Read the model definition and answer for the solid it produces. Units are mm, in the model's axes. Coordinates: 2 decimals unless noted, no trailing zeros. Order: outer loops, then holes, each group sorted by start corner. A loop starts at its lowest first (then second) coordinate and runs counter-clockwise, first axis right, second up. Notation, with made-up numbers: (-15, 21) - (2, 21) arc R21 ccw to (2, 34) - close; hole circle Ø3 at (74, 81). An arc over 180 degrees is marked (long way). Use one line per item in the form item = value.
Autodesk Inventor part; units mm, degrees
ref_plane "Work Plane1" through (0, 12, 0) normal (0, 1, 0) x (-1, 0, 0)
ref_plane "YZ Plane" through (0, 0, 0) normal (1, 0, 0) x (0, 1, 0)
ref_plane "XY Plane" through (0, 0, 0) normal (0, 0, 1) x (1, 0, 0)
sketch "Sketch1" plane through (0, 0, 0) normal (0, 0, 1) x (1, 0, 0)
  arc A0 (0, -12) -> (0, 12) centre (0, 0) ccw
  line L0 (0, 12) -> (0, -12)
  dimension "d0" = 24
revolve "Revolution1" add sketch "Sketch1" angle 360 about axis through (0, 12, 0) along (0, -1, 0)
sketch "Sketch2" plane through (0, 0, 0) normal (0, 1, 0) x (-1, 0, 0)
  circle A0 centre (0, 0) radius 3.175
  dimension "d2" = 6.35
extrude "Extrusion1" cut sketch "Sketch2" along normal through all both and the other way through all
ref_plane "Work Plane1" through (0, 12, 0) normal (0, 1, 0) x (-1, 0, 0)
sketch "Sketch3" plane through (0, 12, 0) normal (0, 1, 0) x (-1, 0, 0)
  circle A0 centre (0, 0) radius 12
extrude "Extrusion2" cut sketch "Sketch3" against normal blind 3
mirror "Mirror1" about plane through (0, 0, 0) normal (0, 1, 0) of "Extrusion2"
properties part number "shifter ball"
(1) Section D-D, the plane z = -9 is taken. Write down the section's boundary in (x, y).
Answer list:
outline = circle Ø15.87 at (0, 0)
(2) Section C-C, the plane y = -1.75 is taken. Write down the section's boundary in (x, z) (3 decimals), then the cut area to 3 significant figures.
Answer list:
outline = circle Ø23.743 at (0, 0); hole circle Ø6.35 at (0, 0)
area = 411 mm2
(3) The mould has two halves that part along Z. Classify faces 1 (the flat face through (3.4, -9, 0.1)), 2 (the cylindrical face through (0.69, 0.13, -3.1)): +Z half, -Z half, draft (parallel to the pull), parting line (faces both ways), or undercut.
Answer list:
face_1 = draft
face_2 = undercut
(4) Section A-A, the plane x = 0 is taken. Write down the section's boundary in (y, z) (3 decimals).
Answer list:
outline = (-9, -7.937) arc R12 ccw to (9, -7.937) - (9, -3.175) - (-9, -3.175) - close; (-9, 3.175) - (9, 3.175) - (9, 7.937) arc R12 ccw to (-9, 7.937) - close
(5) Straight lines are drawn through the part: L1, parallel to X at y = 2.75, z = 2.25; L2, parallel to Z at x = 0, y = 4.5 (3 decimals); L3, parallel to Z at x = 1.75, y = -2. For each, find the intervals that lie inside material, in ascending order.
Answer list:
L1 = -11.46 to -2.24, 2.24 to 11.46
L2 = -11.124 to -3.175, 3.175 to 11.124
L3 = -11.7 to -2.65, 2.65 to 11.7
(6) Section B-B, the plane z = 0 is taken. Write down the section's boundary in (x, y) (3 decimals).
Answer list:
outline = (-7.937, -9) - (-3.175, -9) - (-3.175, 9) - (-7.937, 9) arc R12 ccw to start; (3.175, -9) - (7.937, -9) arc R12 ccw to (7.937, 9) - (3.175, 9) - close
(7) Given pin 1 Ø10 at (y, z) = (-4, -2) entering from -X; pin 2 Ø10 at (y, z) = (5.5, -6.5) entering from +X; pin 3 Ø1 at (x, y) = (4, 4) entering from -Z, each flat-ended and moving along its own axis, determine where each tip first touches the part or whether it passes through.
Answer list:
pin_1 = -12
pin_2 = 11.47
pin_3 = -10.84
